Study the drawing (mm; zero at the part's minimum x, y, z) and answer. Coordinates: 2 decimals unless noted, no trailing zeros. Write each loop counter-clockwise with the first axis right and the second up, starting at its lowest first coordinate (ties: lowest second). Pieces come first, ordered by that corner, then holes. Notation, with made-up numbers: M 40.5,-22.5 L 53.5,-22.5 A34 ccw 53.5,9.5 Z; hole C 46,3 d8. An arc over 180 degrees is marked long. Answer as CSV lines item,"result". Start each with the question number.
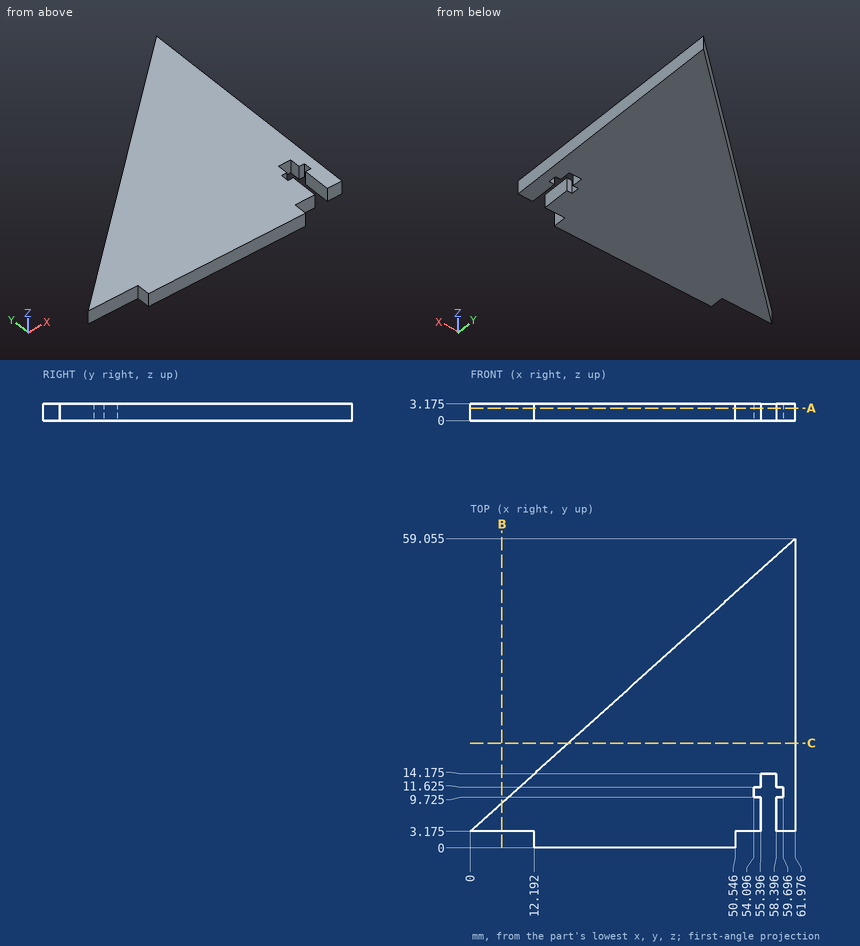
1) The part is cut by section A-A (z = 2.4). Determine the outline of the cut face in (x, y) (3 decimals).
2) Each of these flat-tipped pins is pushed along its axis until it touches: P1, Ø1, axis at x = 61, z = 1, coming from the -Y side (3 decimals); P2, Ø1.6, axis at y = 8, z = 2, coming from the -X side; P3, Ø10, axis at x = 6.5, y = 13.5, coming from the -Z side; P4, Ø0.7, axis at x = 54.5, z = 1, coming from the +Y side. Where does it stop, or does it pass through?
3) The part is cut by section B-B (x = 6). Determine the outline of the cut face in (y, z) (3 decimals).
4) Find the intervals of material crossed by line 1 (X direction, y = 6, z = 2.05); line 2 (X direction, y = 7.5, z = 0.95); line 3 (Y direction, x = 59, z = 0.3) (3 decimals), in increasing order. Write a range as from..to.
5) The part is cut by section C-C (y = 20). Determine the outline of the cut face in (x, z) (3 decimals), then the cut area to 3 significant figures.
Completed:
1,outline,"M 0,3.175 L 12.192,3.175 L 12.192,0 L 50.546,0 L 50.546,3.175 L 55.396,3.175 L 55.396,9.725 L 54.096,9.725 L 54.096,11.625 L 55.396,11.625 L 55.396,14.175 L 58.396,14.175 L 58.396,11.625 L 59.696,11.625 L 59.696,9.725 L 58.396,9.725 L 58.396,3.175 L 61.976,3.175 L 61.976,59.055 Z"
2,P1,"y = 3.175"
2,P2,"x = 4.46"
2,P3,"z = 0"
2,P4,"y = 52.63"
3,outline,"M 3.175,0 L 8.585,0 L 8.585,3.175 L 3.175,3.175 Z"
4,line 1,"3.13..55.4, 58.4..61.98"
4,line 2,"4.8..55.4, 58.4..61.98"
4,line 3,"3.175..9.725, 11.625..56.372"
5,outline,"M 18.66,0 L 61.976,0 L 61.976,3.175 L 18.66,3.175 Z"
5,area,"138 mm²"
